Part model, mm, in its own coordinate system. Give positions to 0.01 mm unless a question says otherwise; leave off trailing zeros. Write each loop counter-clockwise with the first axis right and the second up, starting at its lowest first coordinate (ties: lowest second). Pieces come first, ordered by that corner, then holes. Notation, with made-up numbers: M 33.25,38 L 89.25,38 A17 cw 89.25,43 Z; hole C 85,17 d10. An arc over 180 degrees is marked long. Answer as CSV lines item,"result". Start each with the question number.
1) Mould opens along X. For faces 1 (the cylindrical face through (58.544, -13.137, 15.21)), 2 (the flat face through (-8.717, -35.589, 15.21)), 3 (the flat face through (14, 1, 30)), 4 (the cylindrical face through (-9.764, 74.362, 14.93)) say: pulls with the +X half, pulls with the -X half, needs draft (parallel to the pull), parting line crosses it, or undercut.
2) Slice it at B-B, the plane y = 0. Give the cut face in (x, z).
3) Pin check, flat tips, straight feed: pin 1 Ø5 at (x, z) = (-8, 6) entering from +Y; pin 2 Ø12 at (x, z) = (-59, 7) entering from +Y; pin 3 Ø4 at (y, z) = (-50.5, 24.5) entering from +X. Stop position of each tip, or through.
4) Slice it at A-A, the plane z = 23.5. Give the number of separate pieces and of enclosed holes in the cut face, plus the area to 3 significant figures.
5) Wall check: line 1 along Y through (x, z) = (41, 28); line 2 along Y through (x, z) = (-45.5, 23.5); line 3 along Y through (x, z) = (-21.5, 8). Give the ranges that are in metal, low to high. Write a range as from..to.
```python
from build123d import *

# Parameters (mm, degrees)
SKETCH1_R           = 75
SKETCH1_R_2         = 10
BOSS_EXTRUDE1_DEPTH = 30
CUT_EXTRUDE1_DEPTH  = 111.227038425
FILLET1_R           = 10
CIRPATTERN1_COUNT   = 7


with BuildPart() as part:
    # Sketch1 → Boss-Extrude1 (new body)
    with BuildSketch(Plane.XY):
        Circle(SKETCH1_R)
        Circle(SKETCH1_R_2, mode=Mode.SUBTRACT)
    extrude(amount=BOSS_EXTRUDE1_DEPTH)

    # Sketch2 → Cut-Extrude1 (cut, through all)
    with BuildSketch(Plane.XY.offset(30)):
        with BuildLine():
            Line((0, 15), (-15.39090645, 57.286167935))
            ThreePointArc((-15.39090645, 57.286167935), (0, 60), (15.39090645, 57.286167935))
            Line((15.39090645, 57.286167935), (0, 15))
        make_face()
    cut_extrude1 = extrude(amount=-CUT_EXTRUDE1_DEPTH, mode=Mode.SUBTRACT)

    # Fillet1
    fillet1_edges = [part.edges().sort_by_distance(p)[0] for p in [
        (-75, 0, 0),
        (-75, 0, 30),
    ]]
    fillet(fillet1_edges, radius=FILLET1_R)

    # CirPattern1: Cut-Extrude1 ×7 about axis
    cirpattern1_axis = Axis((0, 0, 0), (0, 0, 1))
    for i in range(1, CIRPATTERN1_COUNT):
        add(cut_extrude1.rotate(cirpattern1_axis, i * 360 / CIRPATTERN1_COUNT), mode=Mode.SUBTRACT)


solid = part.part
```
Found:
1,face 1,"undercut"
1,face 2,"undercut"
1,face 3,"needs draft"
1,face 4,"parting line crosses it"
2,outline,"M -75,10 A10 ccw -65,0 L -59.5,0 L -59.5,30 L -65,30 A10 ccw -75,20 Z; M -41.26,0 L -10,0 L -10,30 L -41.26,30 Z; M 10,0 L 41.26,0 L 41.26,30 L 10,30 Z; M 59.5,0 L 65,0 A10 ccw 75,10 L 75,20 A10 ccw 65,30 L 59.5,30 Z"
3,pin 1,"y = 74.53"
3,pin 2,"y = 52.72"
3,pin 3,"x = 56.14"
4,separate pieces,"1"
4,enclosed holes,"8"
4,area,"12,100 mm²"
5,line 1,"-57.97..-20.37, -0.03..19.19, 43.53..57.97"
5,line 2,"-58.82..-23.28, 0.53..20.7, 39.09..58.82"
5,line 3,"-71.64..-55.94, -28.14..-7.78, -2.48..12.64, 25.34..71.64"
